Geometry check sheet. Reference: the model listing, model coordinates, mm. Face numbers are marked on the shaded views. A direction names the side the tool comes from. Round coordinates to 2 decimals unless told otherwise and drop trailing zeros. Loops run counter-clockwise (first coordinate to the right, second up) from the corner with the lowest first, then second, coordinate; pieces in that order, holes last. Notation, with made-up numbers: (-12.75, 0) - (34.25, 0) arc R17 cw to (34.25, 24) - close; hole circle Ø11 at (-33, -18.5). An arc over 180 degrees is marked (long way). Answer as CSV lines item,"result". Start each with the question number.
1) Cross-section at A-A on z = -2. Record the boundary of the cut face in (x, y) (3 decimals).
2) Thickness scan on line 1 along X through (y, z) = (3, 0) (3 decimals); line 2 along X through (y, z) = (-18, 0.5) (3 decimals); line 3 along Y through (x, z) = (12, -2). Record the ranges inside material, lowest first.
3) Cross-section at B-B on y = 8.5. Record the boundary of the cut face in (x, z) (3 decimals), and give its area (3 significant figures).
4) Depth check by flat-ended pin: P1, Ø1.9, axis at y = 23, z = 1, coming from the -X side (3 decimals); P2, Ø1.9, axis at y = -13, z = 0.5, coming from the -X side (3 decimals); P3, Ø1.5, axis at x = -9.5, y = 17, coming from the +Z side. Enter the tip coordinate at first touch or a pass-through.
5) Access from +Z, -Z, +X, -X, +Y, -Y to the whole of each face (thin tool, end or side, straight path). Record for the marked faces 1 and 2.
from build123d import *

# Parameters (mm, degrees)
F0_W     = 6.35
F0_H     = 6.35
F1_DEPTH = 25.4
F3_DEPTH = 50.8
F4_R     = 3.175
F5_DEPTH = 50.8


with BuildPart() as f1:
    # F0 (on Front) → F1 (new body, symmetric)
    with BuildSketch(Plane.XZ):
        Rectangle(F0_W, F0_H)
    extrude(amount=F1_DEPTH, both=True)

    # F2 (on face) → F3 (join)
    with BuildSketch(Plane.YZ.offset(3.175)):
        with BuildLine():
            ThreePointArc((-19.05, -3.175), (-16.8049359697, -2.2450640303), (-15.875, 0))
            ThreePointArc((-15.875, 0), (-16.8049359657, 2.2450640262), (-19.0499999885, 3.175))
            ThreePointArc((-19.0499999885, 3.175), (-22.225, 5.7e-09), (-19.05, -3.175))
        make_face()
    extrude(amount=F3_DEPTH)

    # F4 (on face) → F5 (join)
    with BuildSketch(Plane(origin=(-3.175, 0, 0), x_dir=(0, -1, 0), z_dir=(-1, 0, 0))):
        with Locations((-19.05, 0)):
            Circle(F4_R)
    extrude(amount=F5_DEPTH)


solid = f1.part
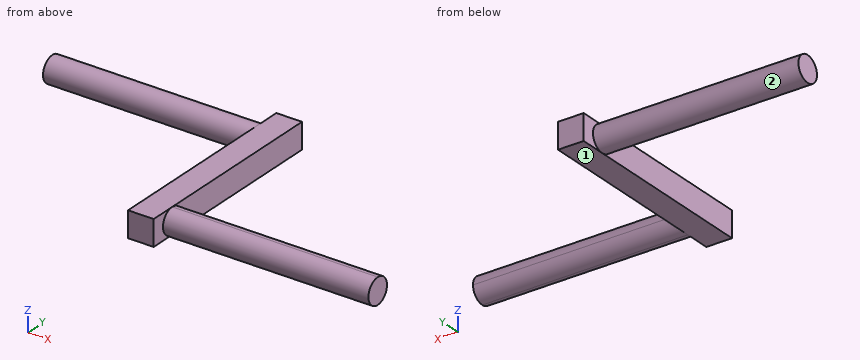
Answer block:
1,outline,"(-53.975, 16.584) - (-3.175, 16.584) - (-3.175, -25.4) - (3.175, -25.4) - (3.175, -21.516) - (53.975, -21.516) - (53.975, -16.584) - (3.175, -16.584) - (3.175, 25.4) - (-3.175, 25.4) - (-3.175, 21.516) - (-53.975, 21.516) - close"
2,line 1,"x = -3.175 to 3.175"
2,line 2,"x = -3.175 to 53.975"
2,line 3,"y = -21.52 to -16.58"
3,outline,"(-3.175, -3.175) - (3.175, -3.175) - (3.175, 3.175) - (-3.175, 3.175) - close"
3,area,"40.3 mm^2"
4,P1,"stops at x = -53.975"
4,P2,"stops at x = -3.175"
4,P3,"stops at z = 2.9"
5,face 1,"-Z, +X, -X, +Y, -Y"
5,face 2,"-X"
